Check sheet for the modelled part. Datum: model origin and axes. Units: mm. Face numbers are marked on the shaded views. A direction names the side the tool comes from. Round coordinates to 2 decimals unless told otherwise and drop trailing zeros. Loops run counter-clockwise (first coordinate to the right, second up) from the corner with the lowest first, then second, coordinate; pieces in that order, holes last. Notation, with made-up numbers: M -24,89.5 L 17,89.5 A14 ccw 17,97.5 Z; hole C 47,1.5 d8. An arc over 180 degrees is marked long. Write item = value, one per line. Start each with the question number.
(1) Cross-section at B-B on z = 57.15. Record the boundary of the cut face in (x, y) (3 decimals), plus the area to 3 significant figures.
(2) Cross-section at D-D on z = -3. Record the boundary of the cut face in (x, y), plus the area to 3 significant figures.
(3) Cross-section at A-A on x = -38.1. Record the boundary of the cut face in (y, z) (3 decimals), plus the area to 3 significant figures.
(4) Scan lines: L1, parallel to Z at x = 38.1, y = 1.2 (3 decimals); L2, parallel to X at y = 0.7, z = 57.15 (3 decimals); L3, parallel to Z at x = 22, y = 8.75 (3 decimals). Record each from-to range of solid material in increasing order. Write a range as from..to.
(5) Set-up check for the marked faces 1, 2 and 3: record each of +Z, -Z, +X, -X, +Y, -Y from which the full face is reachable in a straight line by a thin tool's end or side.
(6) Go/stop test with flat-tipped pins: P1, Ø4, axis at x = 4, y = 7.5, coming from the -Z side; P2, Ø8.5, axis at x = -38.1, z = -57.15, coming from the +Y side; P3, Ø1.5, axis at x = 21.5, y = 12, coming from the +Z side; P4, Ø4, axis at x = -38.1, z = 57.15, coming from the -Y side. Record where each tip stops, or that it passes through.
(7) Cross-section at C-C on x = -13.5. Record the boundary of the cut face in (y, z) (3 decimals).
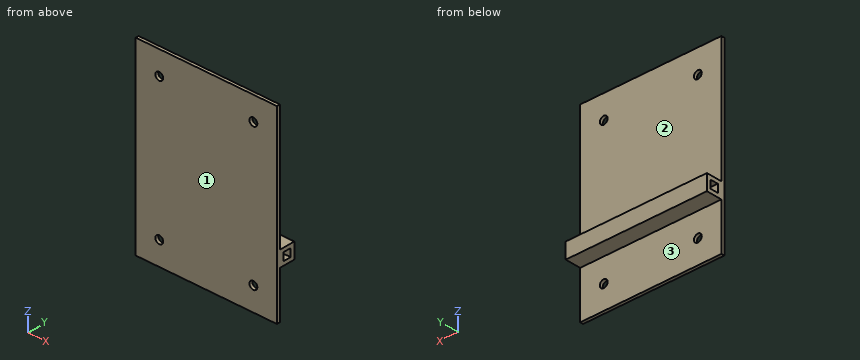
from build123d import *

# Parameters (mm, degrees)
SKETCH1_W           = 114.3
SKETCH1_H           = 152.4
BOSS_EXTRUDE1_DEPTH = 2.54
SKETCH2_W           = 114.3
SKETCH2_H           = 12.7
BOSS_EXTRUDE2_DEPTH = 12.7
SKETCH3_W           = 6.35
SKETCH3_H           = 6.35
CUT_EXTRUDE1_DEPTH  = 115.3
SKETCH4_R           = 3.175
CUT_EXTRUDE2_DEPTH  = 3.54


with BuildPart() as part:
    # Sketch1 → Boss-Extrude1 (new body)
    with BuildSketch(Plane(origin=(0, 0, 0), x_dir=(1, 0, 0), z_dir=(0, 1, 0))):
        Rectangle(SKETCH1_W, SKETCH1_H)
    extrude(amount=BOSS_EXTRUDE1_DEPTH)

    # Sketch2 → Boss-Extrude2 (add)
    with BuildSketch(Plane(origin=(0, 2.54, 0), x_dir=(1, 0, 0), z_dir=(0, 1, 0))):
        with Locations((0, 31.75)):
            Rectangle(SKETCH2_W, SKETCH2_H)
    extrude(amount=BOSS_EXTRUDE2_DEPTH)

    # Sketch3 → Cut-Extrude1 (cut, through all)
    with BuildSketch(Plane.ZY.offset(57.15)):
        with Locations((-31.75, 8.89)):
            Rectangle(SKETCH3_W, SKETCH3_H)
    extrude(amount=-CUT_EXTRUDE1_DEPTH, mode=Mode.SUBTRACT)

    # Sketch4 → Cut-Extrude2 (cut, through all)
    with BuildSketch(Plane(origin=(0, 2.54, 0), x_dir=(1, 0, 0), z_dir=(0, 1, 0))):
        with Locations((-38.1, 57.15)):
            Circle(SKETCH4_R)
        with Locations((38.1, 57.15)):
            Circle(SKETCH4_R)
        with Locations((-38.1, -57.15)):
            Circle(SKETCH4_R)
        with Locations((38.1, -57.15)):
            Circle(SKETCH4_R)
    extrude(amount=-CUT_EXTRUDE2_DEPTH, mode=Mode.SUBTRACT)


solid = part.part
Result:
q1.outline = M -57.15,0 L -41.275,0 L -41.275,2.54 L -57.15,2.54 Z; M -34.925,0 L 34.925,0 L 34.925,2.54 L -34.925,2.54 Z; M 41.275,0 L 57.15,0 L 57.15,2.54 L 41.275,2.54 Z
q1.area = 258 mm^2
q2.outline = M -57.15,0 L 57.15,0 L 57.15,2.54 L -57.15,2.54 Z
q2.area = 290 mm^2
q3.outline = M 0,-76.2 L 2.54,-76.2 L 2.54,-60.325 L 0,-60.325 Z; M 0,-53.975 L 2.54,-53.975 L 2.54,-38.1 L 15.24,-38.1 L 15.24,-25.4 L 2.54,-25.4 L 2.54,53.975 L 0,53.975 Z; M 0,60.325 L 2.54,60.325 L 2.54,76.2 L 0,76.2 Z; hole M 5.715,-34.925 L 12.065,-34.925 L 12.065,-28.575 L 5.715,-28.575 Z
q3.area = 476 mm^2
q4.L1 = -76.2..-60.325, -53.975..53.975, 60.325..76.2
q4.L2 = -57.15..-41.275, -34.925..34.925, 41.275..57.15
q4.L3 = -38.1..-34.925, -28.575..-25.4
q5.face_1 = +Z, -Z, +X, -X, -Y
q5.face_2 = +Z, +X, -X, +Y
q5.face_3 = -Z, +X, -X, +Y
q6.P1 = -38.1
q6.P2 = 2.54
q6.P3 = -25.4
q6.P4 = through
q7.outline = M 0,-76.2 L 2.54,-76.2 L 2.54,-38.1 L 15.24,-38.1 L 15.24,-25.4 L 2.54,-25.4 L 2.54,76.2 L 0,76.2 Z; hole M 5.715,-34.925 L 12.065,-34.925 L 12.065,-28.575 L 5.715,-28.575 Z
